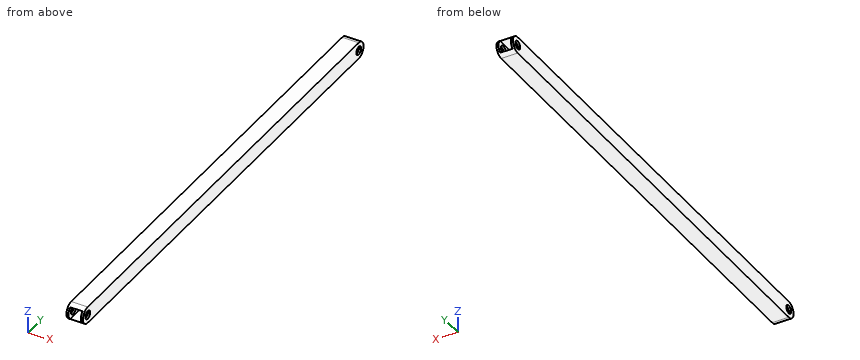
Autodesk Inventor part; units mm, degrees
ref_plane "YZ Plane" through (0, 0, 0) normal (1, 0, 0) x (0, 1, 0)
ref_plane "XZ Plane" through (0, 0, 0) normal (0, 1, 0) x (-1, 0, 0)
ref_plane "XY Plane" through (0, 0, 0) normal (0, 0, 1) x (1, 0, 0)
sketch "Sketch1" plane through (0, 0, 0) normal (0, 1, 0) x (-1, 0, 0)
  line L0 (0, 0) -> (12.7, 0)
  line L1 (12.7, 0) -> (12.7, -12.7)
  line L2 (12.7, -12.7) -> (0, -12.7)
  line L3 (0, -12.7) -> (0, 0)
  line L4 (11.1252, -1.5748) -> (1.5748, -1.5748)
  line L5 (1.5748, -1.5748) -> (1.5748, -11.1252)
  line L6 (1.5748, -11.1252) -> (11.1252, -11.1252)
  line L7 (11.1252, -11.1252) -> (11.1252, -1.5748)
  line L8 (6.35, -1.5748) -> (6.35, 0) construction
  line L9 (1.5748, -6.35) -> (0, -6.35) construction
  dimension "d0" = 12.7
  dimension "d1" = 1.5748
extrude "Extrusion1" add sketch "Sketch1" along normal blind 369.57
sketch "Sketch2" plane through (0, 0, 0) normal (1, 0, 0) x (0, 0, -1)
  line L0 (0, 0) -> (12.7, 0) construction
  line L1 (6.35, 0) -> (6.35, 369.57) construction
  line L2 (0, 369.57) -> (12.7, 369.57) construction
  line L3 (0, 0) -> (0, 369.57) construction
  line L4 (0, 184.785) -> (12.7, 184.785) construction
  circle A0 centre (6.35, 6.35) radius 3.175
  circle A1 centre (6.35, 363.22) radius 3.175
  dimension "d4" = 6.35
  dimension "d5" = 356.87
extrude "Extrusion2" cut sketch "Sketch2" against normal through all
fillet "Fillet1" radius 6.35 4 edges at (-6.35, 369.57, 0) (-6.35, 369.57, -12.7) (-6.35, 0, 0) (-6.35, 0, -12.7)
properties part number "Tie Rod"
The model under review builds one solid part; all positions refer to its coordinate system, in mm. Round coordinates to 2 decimals unless told otherwise and drop trailing zeros. Loops run counter-clockwise (first coordinate to the right, second up) from the corner with the lowest first, then second, coordinate; pieces in that order, holes last. Notation, with made-up numbers: M -13,19.5 L 46,19.5 A16 cw 46,39.5 Z; hole C -22,81 d4. An arc over 180 degrees is marked long. Answer as CSV lines item,"result". Start each with the question number.
Item 1: Consider section B-B (z = -6.35). Write out the cut boundary in (x, y) (3 decimals).
Item 2: Consider section C-C (y = 92). Write out the cut boundary in (x, z), then the cut area to 3 significant figures.
Item 3: Insertion check: P1, Ø4, axis at y = 363.22, z = -6.35, coming from the +X side. The pin has a flat end and moves straight along its axis. Give the tip position at first contact, or say it passes through.
Item 4: Wall thickness on line 1 (Y direction, x = -12.2, z = -6.35) (3 decimals); line 2 (Z direction, x = -4, y = 285.5): over which ranges is each line inside the solid? List them lowest first. Write a range as [from, to].
Item 5: Consider section A-A (x = -4.5). Write out the cut boundary in (y, z).
Answer:
1,outline,"M -12.7,0 L -11.125,0 L -11.125,3.175 L -12.7,3.175 Z; M -12.7,9.525 L -11.125,9.525 L -11.125,360.045 L -12.7,360.045 Z; M -12.7,366.395 L -11.125,366.395 L -11.125,369.57 L -12.7,369.57 Z; M -1.575,0 L 0,0 L 0,3.175 L -1.575,3.175 Z; M -1.575,9.525 L 0,9.525 L 0,360.045 L -1.575,360.045 Z; M -1.575,366.395 L 0,366.395 L 0,369.57 L -1.575,369.57 Z"
2,outline,"M -12.7,-12.7 L 0,-12.7 L 0,0 L -12.7,0 Z; hole M -11.13,-11.13 L -1.57,-11.13 L -1.57,-1.57 L -11.13,-1.57 Z"
2,area,"70.1 mm^2"
3,P1,"passes through"
4,line 1,"y = [0, 3.175], [9.525, 360.045], [366.395, 369.57]"
4,line 2,"z = [-12.7, -11.13], [-1.57, 0]"
5,outline,"M 2.16,-11.13 A6.35 ccw 6.35,-12.7 L 363.22,-12.7 A6.35 ccw 367.41,-11.13 Z; M 2.16,-1.57 L 367.41,-1.57 A6.35 ccw 363.22,0 L 6.35,0 A6.35 ccw Z"
